Source: CAD feature listing. Evaluate the final solid. Frame: model axes, mm. Face numbers are marked on the shaded views. Coordinates: 2 decimals unless noted, no trailing zeros. Write each loop counter-clockwise with the first axis right and the second up, starting at its lowest first coordinate (ties: lowest second). Pieces come first, ordered by that corner, then holes. Notation, with made-up numbers: (69.25, 11.25) -> (86.25, 11.25) arc R3 ccw to (86.25, 16.25) -> close; hole circle Ø10 at (17.25, -32). An arc over 180 degrees is marked (long way). One line per item, written item: value. Start each with the question number.
1. Section query C-C, the plane z = -53. Output: boundary loops of the cut face in (x, y).
2. Mould query, pull axis X, two halves, no side actions, for the marked faces 1, 2, 3 and 4. Classes: released by +X, released by -X, zero draft, split by the parting line, or undercut.
3. Section query B-B, the plane y = 87.5. Output: boundary loops of the cut face in (x, z), and give its area (4 significant figures).
4. Line query: line 1 (X direction, y = 23, z = 151.5); line 2 (Y direction, x = 192, z = -75); line 3 (Y direction, x = 155.75, z = 87). Output: solid intervals per line, ascending.
5. Section query D-D, the plane y = 185. State how many separate pieces and enclosed holes the cut face has, and give its area (3 significant figures).
6. Section query A-A, the plane z = 87. Output: boundary loops of the cut face in (x, y).
7. First-contact query: P1, Ø8, axis at x = -20, y = 33, coming from the +Z side; P2, Ø4.5, axis at x = -154.5, y = 151, coming from the +Z side. Flat tips, straight axial feed; report the tip coordinate or a pass-through.
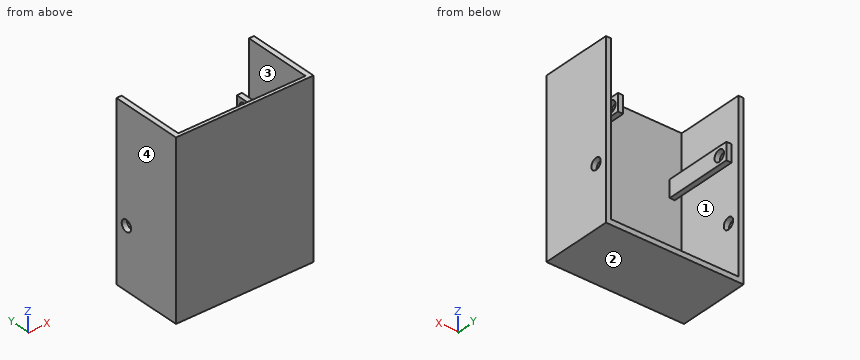
from build123d import *

# Parameters (mm, degrees)
SKETCH3_W               = 400
SKETCH3_H               = 500
BOSS_EXTRUDE1_DEPTH     = 10
BOSS_EXTRUDE3_DEPTH     = 200
CUT_EXTRUDE1_DEPTH      = 517.333225737
CUT_EXTRUDE1_DEPTH_BACK = 517.333225737
SKETCH5_R               = 16.5
SKETCH6_W               = 15
SKETCH6_H               = 50
BOSS_EXTRUDE4_DEPTH     = 200
SKETCH9_R               = 16.5
CUT_EXTRUDE3_DEPTH      = 15
SKETCH10_R              = 16.5
CUT_EXTRUDE4_DEPTH      = 15


with BuildPart() as part:
    # Sketch3 → Boss-Extrude1 (new body)
    with BuildSketch(Plane(origin=(0, 0, 0), x_dir=(1, 0, 0), z_dir=(0, 1, 0))):
        Rectangle(SKETCH3_W, SKETCH3_H)
    extrude(amount=BOSS_EXTRUDE1_DEPTH)

    # Sketch4 → Boss-Extrude3 (add)
    with BuildSketch(Plane(origin=(0, 10, 0), x_dir=(1, 0, 0), z_dir=(0, 1, 0))):
        Polygon((-185, -250), (-185, -235), (-185, 235), (185, 235), (185, -235), (185, -250), (200, -250), (200, 250), (-200, 250), (-200, -250), align=None)
    extrude(amount=BOSS_EXTRUDE3_DEPTH)

    # Sketch5 → Cut-Extrude1 (cut, two sides: drawn at the far end of the back side and taken through both)
    with BuildSketch(Plane.ZY.offset(200).offset(-CUT_EXTRUDE1_DEPTH_BACK)):
        with Locations(Location((-75, 175, 0), (0, 0, 180))):
            Circle(SKETCH5_R)
    extrude(amount=CUT_EXTRUDE1_DEPTH + CUT_EXTRUDE1_DEPTH_BACK, mode=Mode.SUBTRACT)

    # Sketch6 → Boss-Extrude4 (add)
    with BuildSketch(Plane(origin=(0, 10, 0), x_dir=(1, 0, 0), z_dir=(0, 1, 0))):
        with Locations((-157.5, -87)):
            Rectangle(SKETCH6_W, SKETCH6_H)
        with Locations((157.5, -87)):
            Rectangle(SKETCH6_W, SKETCH6_H)
    extrude(amount=BOSS_EXTRUDE4_DEPTH)

    # Sketch9 → Cut-Extrude3 (cut)
    with BuildSketch(Plane(origin=(-150, 0, 0), x_dir=(0, 0, -1), z_dir=(1, 0, 0))):
        with Locations((-87, 185)):
            Circle(SKETCH9_R)
    extrude(amount=-CUT_EXTRUDE3_DEPTH, mode=Mode.SUBTRACT)

    # Sketch10 → Cut-Extrude4 (cut)
    with BuildSketch(Plane(origin=(165, 0, 0), x_dir=(0, 0, -1), z_dir=(1, 0, 0))):
        with Locations((-87, 185)):
            Circle(SKETCH10_R)
    extrude(amount=-CUT_EXTRUDE4_DEPTH, mode=Mode.SUBTRACT)


solid = part.part
Computed values:
1. outline: (-200, 0) -> (200, 0) -> (200, 210) -> (185, 210) -> (185, 10) -> (-185, 10) -> (-185, 210) -> (-200, 210) -> close
2. face 1: undercut
2. face 2: zero draft
2. face 3: undercut
2. face 4: released by -X
3. outline: (-200, -250) -> (200, -250) -> (200, 250) -> (185, 250) -> (185, -235) -> (-185, -235) -> (-185, 250) -> (-200, 250) -> close; (-165, 62) -> (-150, 62) -> (-150, 112) -> (-165, 112) -> close; (150, 62) -> (165, 62) -> (165, 112) -> (150, 112) -> close
3. area: 22,050 mm²
4. line 1: x = -200 to -185, 185 to 200
4. line 2: y = 0 to 158.5, 191.5 to 210
4. line 3: y = 0 to 168.5, 201.5 to 210
5. separate pieces: 7
5. enclosed holes: 0
5. area: 20,300 mm²
6. outline: (-200, 0) -> (200, 0) -> (200, 210) -> (185, 210) -> (185, 10) -> (165, 10) -> (165, 168.5) -> (150, 168.5) -> (150, 10) -> (-150, 10) -> (-150, 168.5) -> (-165, 168.5) -> (-165, 10) -> (-185, 10) -> (-185, 210) -> (-200, 210) -> close; (-165, 201.5) -> (-150, 201.5) -> (-150, 210) -> (-165, 210) -> close; (150, 201.5) -> (165, 201.5) -> (165, 210) -> (150, 210) -> close
7. P1: stops at z = -235
7. P2: stops at z = 112
